Geometry check sheet. Reference: the model listing, model coordinates, mm. A direction names the side the tool comes from. Round coordinates to 2 decimals unless told otherwise and drop trailing zeros. Write each loop counter-clockwise with the first axis right and the second up, starting at its lowest first coordinate (ties: lowest second). Pieces come first, ordered by that corner, then holes. Notation, with made-up numbers: M -18,-37 L 3,-37 A11 cw 3,-18 Z; hole C 83,18.25 d6. An arc over 180 degrees is marked long. Use a Markdown table: item, result.
Autodesk Inventor part; units mm, degrees
ref_plane "YZ Plane" through (0, 0, 0) normal (1, 0, 0) x (0, 1, 0)
ref_plane "XZ Plane" through (0, 0, 0) normal (0, 1, 0) x (-1, 0, 0)
ref_plane "XY Plane" through (0, 0, 0) normal (0, 0, 1) x (1, 0, 0)
sketch "Sketch1" plane through (0, 0, 0) normal (0, 0, 1) x (1, 0, 0)
  line L0 (-30, -15) -> (30, -15)
  line L1 (30, -15) -> (30, 15)
  line L2 (30, 15) -> (-30, 15)
  line L3 (-30, 15) -> (-30, -15)
  line L4 (-30, -15) -> (30, 15) construction
  line L5 (30, -15) -> (-30, 15) construction
  point P0 (0, 0)
  dimension "d0" = 60
  dimension "d1" = 30
extrude "Extrusion1" add sketch "Sketch1" along normal blind 10
sketch "Sketch2" plane through (0, 0, 10) normal (0, 0, 1) x (1, 0, 0)
  circle A0 centre (0, 0) radius 10.5
  dimension "d4" = 21
extrude "Extrusion2" cut sketch "Sketch2" against normal blind 5
sketch "Sketch3" plane through (0, 0, 5) normal (0, 0, 1) x (1, 0, 0)
  circle A0 centre (0, 0) radius 8
  dimension "d7" = 16
extrude "Extrusion3" cut sketch "Sketch3" against normal blind 5
sketch "Sketch4" plane through (0, 0, 10) normal (0, 0, 1) x (1, 0, 0)
  point P0 (0, 0)
  point P1 (-24.4767, 0)
  point P2 (24.786, 0)
hole "Hole1" at (-24.4767, 0, 10) at (24.786, 0, 10) direction (0, 0, -1) diameter 6.6 end through all
fillet "Fillet1" radius 1 4 edges at (30, 15, 5) (30, -15, 5) (-30, 15, 5) (-30, -15, 5)
properties part number "CoinCellHolder"
Item 1: Cross-section at B-B, the plane y = 0. Record the cut outline in (x, z).
Outcome:
| item | result |
|---|---|
| outline | M -30,0 L -27.78,0 L -27.78,10 L -30,10 Z; M -21.18,0 L -8,0 L -8,5 L -10.5,5 L -10.5,10 L -21.18,10 Z; M 8,0 L 21.49,0 L 21.49,10 L 10.5,10 L 10.5,5 L 8,5 Z; M 28.09,0 L 30,0 L 30,10 L 28.09,10 Z |
Item 2: Mould release check, pull along Y, two halves, no side actions. Record for faces 3 (the face through (-30, 0, 5)), 4 (the face through (-1.73, -7.81, 2.54)), 5 (the face through (0, -15, 5)): +Y half, -Y half, draft (parallel to the pull), parting line (faces both ways), or undercut.
Outcome:
| item | result |
|---|---|
| face 3 | draft |
| face 4 | undercut |
| face 5 | -Y half |
Item 3: Access from +Z, -Z, +X, -X, +Y, -Y to the whole of each face (thin tool, end or side, straight path). Record for faces 1 (the face through (10, 3.2, 7.5)), 2 (the face through (-21.255, 0.715, 4.93)).
Outcome:
| item | result |
|---|---|
| face 1 | +Z |
| face 2 | +Z, -Z |
Item 4: Cross-section at C-C, the plane z = 7.25. Record the cut outline in (x, y), and give its area (3 significant figures).
Outcome:
| item | result |
|---|---|
| outline | M -30,-14 A1 ccw -29,-15 L 29,-15 A1 ccw 30,-14 L 30,14 A1 ccw 29,15 L -29,15 A1 ccw -30,14 Z; hole C -24.48,0 d6.6; hole C 0,0 d21; hole C 24.79,0 d6.6 |
| area | 1,380 mm2 |
Item 5: Cross-section at D-D, the plane y = 4. Record the cut outline in (x, z), and give its area (3 significant figures).
Outcome:
| item | result |
|---|---|
| outline | M -30,0 L -6.93,0 L -6.93,5 L -9.71,5 L -9.71,10 L -30,10 Z; M 6.93,0 L 30,0 L 30,10 L 9.71,10 L 9.71,5 L 6.93,5 Z |
| area | 434 mm2 |
Item 6: Cross-section at A-A, the plane x = 0. Record the cut outline in (y, z).
Outcome:
| item | result |
|---|---|
| outline | M -15,0 L -8,0 L -8,5 L -10.5,5 L -10.5,10 L -15,10 Z; M 8,0 L 15,0 L 15,10 L 10.5,10 L 10.5,5 L 8,5 Z |
Item 7: Material ranges on line 1 along X through (y, z) = (0.5, 8.5); line 2 along X through (y, z) = (-2, 7); line 3 along X through (y, z) = (4.5, 6.25), recorded low to high. Write a range as from..to.
Outcome:
| item | result |
|---|---|
| line 1 | x = -30..-27.74, -21.21..-10.49, 10.49..21.52, 28.05..30 |
| line 2 | x = -30..-27.1, -21.85..-10.31, 10.31..22.16, 27.41..30 |
| line 3 | x = -30..-9.49, 9.49..30 |
